```python
from build123d import *

# Parameters (mm, degrees)
BOSS_EXTRUDE1_DEPTH = 1.5875
FILLET1_R           = 127
FILLET2_R           = 25.4
SKETCH2_W           = 3.302
SKETCH2_H           = 12.7
SKETCH2_W_2         = 3.3782
CUT_EXTRUDE1_DEPTH  = 4.175


with BuildPart() as part:
    # Sketch1 → Boss-Extrude1 (new body, symmetric)
    with BuildSketch(Plane.XY):
        with BuildLine():
            Line((0, -97.5), (0, -91.458484162))
            Line((0, -91.458484162), (0, -84.854484162))
            Line((0, -84.854484162), (0, -82.26))
            ThreePointArc((0, -82.26), (1.897011907, -83.568972596), (3.81, -84.854484162))
            ThreePointArc((3.81, -84.854484162), (46.908813116, -106.039615985), (93.98, -115.559115329))
            ThreePointArc((93.98, -115.559115329), (339.07784145, -114.653396415), (582.298149945, -84.360596188))
            Line((582.298149945, -84.360596188), (583.523082908, -97.001384899))
            Line((583.523082908, -97.001384899), (550.289320925, -104.328123724))
            Line((550.289320925, -104.328123724), (527.710073756, -120.138282799))
            Line((527.710073756, -120.138282799), (110.986490966, -152.337740244))
            Line((110.986490966, -152.337740244), (93.98, -128.27))
            ThreePointArc((93.98, -128.27), (45.056564108, -118.790242286), (0, -97.5))
        make_face()
    extrude(amount=BOSS_EXTRUDE1_DEPTH, both=True)

    # Fillet1
    fillet1_edges = [part.edges().sort_by_distance(p)[0] for p in [
        (550.289320925, -104.328123724, -0.79375),
    ]]
    fillet(fillet1_edges, radius=FILLET1_R)

    # Fillet2
    fillet2_edges = [part.edges().sort_by_distance(p)[0] for p in [
        (93.98, -128.27, 0.79375),
    ]]
    fillet(fillet2_edges, radius=FILLET2_R)

    # Sketch2 → Cut-Extrude1 (cut, through all)
    with BuildSketch(Plane.XY.offset(1.5875)):
        with Locations((1.651, -84.72524711)):
            Rectangle(SKETCH2_W, SKETCH2_H)
        with Locations((93.98, -113.91339143)):
            Rectangle(SKETCH2_W_2, SKETCH2_H)
        Polygon((190.965218572, -126.030176605), (194.342678534, -125.959469873), (194.076863752, -113.262251969), (190.69940379, -113.332958701), align=None)
        Polygon((289.697985722, -121.153429558), (293.07306112, -121.008166691), (292.800010619, -114.664040004), (289.424935222, -114.80930287), align=None)
    extrude(amount=-CUT_EXTRUDE1_DEPTH, mode=Mode.SUBTRACT)


solid = part.part
```
Design review of the part built by this model. Coordinates are the model's own, in mm. A direction names the side the tool comes from. Give positions to 0.01 mm unless a question says otherwise; leave off trailing zeros. Write each loop counter-clockwise with the first axis right and the second up, starting at its lowest first coordinate (ties: lowest second). Pieces come first, ordered by that corner, then holes. Notation, with made-up numbers: (-21.5, 57.25) - (0.5, 57.25) arc R20 ccw to (0.5, 85.25) - close; hole circle Ø5 at (-24, -5.5). An arc over 180 degrees is marked (long way). Return JSON: item names as keys, results as strings. Group by question number.
(1) Machinability: for faces 1 (the flat face through (293, -128, 1.588)), 2 (the cylindrical face through (436.16, -106.12, 0.02)), which of the approach directions +Z, -Z, +X, -X, +Y, -Y give a long, thin tool a straight path to every point of the face, cutting with its end or side? Answer none if there is none.
(2) We need section B-B, the plane y = -104. Give the boundary of the cut face in (x, z), then the cut area to 3 significant figures.
(3) We need section D-D, the plane y = -133. Give the boundary of the cut face in (x, z).
(4) We need section A-A, the plane z = -0.35. Give the boundary of the cut face in (x, y), then the cut area to 3 significant figures.
(5) Insertion check: pin 1 (1 mm diameter, centred on x = 478, z = 0, fed in from +Y); pin 2 (1.5 mm diameter, centred on x = 456.5, z = 0.5, fed in from +Y); pin 3 (1 mm diameter, centred on y = -118, z = -0.5, fed in from +X). Each pin has a flat end and moves straight along its axis. Give the tip position at first contact, or say it passes through.
(6) To check wall thickness, follow probe 1 along Y at (x, z) = (270, -0.8); probe 2 along Y at (x, z) = (178.5, -0.7). State the ranges of each line that lie inside material, in increasing order.
(7) We need section C-C, the plane x = 257.5. Give the boundary of the cut face in (y, z).
Reported:
{
 "1": {"face 1": "+Z, +X, -X, +Y, -Y", "face 2": "+Z, -Z, +Y"},
 "2": {"outline": "(10.98, -1.59) - (41.22, -1.59) - (41.22, 1.59) - (10.98, 1.59) - close; (454.33, -1.59) - (557.73, -1.59) - (557.73, 1.59) - (454.33, 1.59) - close", "area": "424 mm2"},
 "3": {"outline": "(96.3, -1.59) - (361.25, -1.59) - (361.25, 1.59) - (96.3, 1.59) - close"},
 "4": {"outline": "(0, -97.5) arc R199.83 ccw to (83.04, -127.24) arc R25.4 cw to (100.71, -137.8) - (110.99, -152.34) - (527.71, -120.14) - (529.53, -118.86) arc R127 cw to (575.03, -98.87) - (583.52, -97) - (582.3, -84.36) arc R2040.06 cw to (292.9, -117.08) - (293.07, -121.01) - (289.7, -121.15) - (289.53, -117.21) arc R2040.06 cw to (194.19, -118.75) - (194.34, -125.96) - (190.97, -126.03) - (190.81, -118.72) arc R2040.06 cw to (95.67, -115.65) - (95.67, -120.26) - (92.29, -120.26) - (92.29, -115.43) arc R187.15 cw to (3.3, -84.52) - (3.3, -91.08) - (0, -91.08) - close", "area": "12,600 mm2"},
 "5": {"pin 1": "stops at y = -100.93", "pin 2": "stops at y = -103.64", "pin 3": "stops at x = 531.52"},
 "6": {"probe 1": "y = -140.05 to -117.89", "probe 2": "y = -147.12 to -118.58"},
 "7": {"outline": "(-141.02, -1.59) - (-118.23, -1.59) - (-118.23, 1.59) - (-141.02, 1.59) - close"}
}
